```python
from build123d import *

# Parameters (mm, degrees)
BOSS_EXTRUDE6_DEPTH     = 13
SKETCH10_W              = 35
SKETCH10_H              = 50
BOSS_EXTRUDE7_DEPTH     = 200
BOSS_EXTRUDE8_DEPTH     = 13
BOSS_EXTRUDE10_DEPTH    = 200
FILLET2_R               = 0.2
FILLET3_R               = 0.2
SKETCH13_W              = 69.491392083
SKETCH13_H              = 95.024424652
SKETCH13_W_2            = 70.992171295
SKETCH13_H_2            = 120
CUT_EXTRUDE1_DEPTH      = 40
CUT_EXTRUDE1_DEPTH_BACK = 40
FILLET4_R               = 2


with BuildPart() as part:
    # Sketch9 → Boss-Extrude6 (new body)
    with BuildSketch(Plane(origin=(54.235591649, 0, 0), x_dir=(1, 0, 0), z_dir=(0, 0, 1))):
        Polygon((26.684813292, -242.858935562), (22.210553706, -242.858935562), (18.123114185, -244.678780887), (15.129250155, -248.003803746), (13.746627905, -252.259077482), (14.214315384, -256.708826606), (16.451445177, -260.583649071), (20.07119722, -263.213552871), (24.447683499, -264.143803746), (28.824169779, -263.213552871), (32.443921821, -260.583649071), (34.681051615, -256.708826606), (35.148739093, -252.259077482), (33.766116844, -248.003803746), (30.772252814, -244.678780887), align=None)
    extrude(amount=BOSS_EXTRUDE6_DEPTH)

    # Sketch10 → Boss-Extrude7 (add)
    with BuildSketch(Plane.XY.offset(13)):
        with Locations((78.683275149, -253.383803746)):
            Rectangle(SKETCH10_W, SKETCH10_H)
    extrude(amount=BOSS_EXTRUDE7_DEPTH)

    # Sketch11 → Boss-Extrude8 (add)
    with BuildSketch(Plane.XY.offset(213)):
        Polygon((78.683275149, -264.143803746), (83.059761428, -263.213552871), (86.679513471, -260.583649071), (88.916643264, -256.708826606), (89.384330743, -252.259077482), (88.001708493, -248.003803746), (85.007844463, -244.678780887), (80.920404942, -242.858935562), (76.446145356, -242.858935562), (72.358705834, -244.678780887), (69.364841804, -248.003803746), (67.982219555, -252.259077482), (68.449907033, -256.708826606), (70.687036827, -260.583649071), (74.306788869, -263.213552871), align=None)
    extrude(amount=BOSS_EXTRUDE8_DEPTH)

    # Sketch12 → Boss-Extrude10 (add)
    with BuildSketch(Plane.XY.offset(213)):
        Polygon((99.546985742, -240.476339651), (99.546985742, -240.976339651), (96.183275149, -240.976339651), (96.183275149, -245.876341177), (99.546985742, -245.876341177), (99.546985742, -246.376341177), (101.738909258, -245.329800525), (101.738909258, -244.726339651), (97.997187134, -244.726339651), (97.496982691, -244.234356535), (97.496982691, -242.626350386), (97.99698111, -242.126341177), (101.738909258, -242.126341177), (101.738909258, -241.524181899), align=None)
    extrude(amount=-BOSS_EXTRUDE10_DEPTH)

    # Fillet2
    fillet2_edges = [part.edges().sort_by_distance(p)[0] for p in [
        (101.738909258, -241.524181899, 113),
        (101.738909258, -242.126341177, 113),
        (97.99698111, -242.126341177, 113),
        (97.496982691, -242.626350386, 113),
        (97.496982691, -244.234356535, 113),
        (97.997187134, -244.726339651, 113),
        (101.738909258, -245.329800525, 113),
    ]]
    fillet(fillet2_edges, radius=FILLET2_R)

    # Fillet3
    fillet3_edges = [part.edges().sort_by_distance(p)[0] for p in [
        (101.738909258, -244.726339651, 113),
    ]]
    fillet(fillet3_edges, radius=FILLET3_R)

    # Sketch13 → Cut-Extrude1 (cut, two sides)
    with BuildSketch(Plane(origin=(0, -240.976339651, 0), x_dir=(1, 0, 0), z_dir=(0, 1, 0))) as cut_extrude1_sk:
        with Locations((130.928971191, -51.487787674)):
            Rectangle(SKETCH13_W, SKETCH13_H)
        with Locations((131.679360797, -187)):
            Rectangle(SKETCH13_W_2, SKETCH13_H_2)
    extrude(amount=CUT_EXTRUDE1_DEPTH, mode=Mode.SUBTRACT)
    extrude(cut_extrude1_sk.sketch, amount=-CUT_EXTRUDE1_DEPTH_BACK, mode=Mode.SUBTRACT)

    # Fillet4
    fillet4_edges = [part.edges().sort_by_distance(p)[0] for p in [
        (96.183275149, -278.383803746, 113),
        (96.183275149, -228.383803746, 113),
        (61.183275149, -228.383803746, 113),
        (61.183275149, -278.383803746, 113),
    ]]
    fillet(fillet4_edges, radius=FILLET4_R)


solid = part.part
```
Here's how the part is built. I have some questions about the finished solid (model axes, mm). A direction names the side the tool comes from. Round coordinates to 2 decimals unless told otherwise and drop trailing zeros. Loops run counter-clockwise (first coordinate to the right, second up) from the corner with the lowest first, then second, coordinate; pieces in that order, holes last.
1. Suppose I cut it at B-B, the plane y = -235.5. Please give me the cut outline in (x, z), and give its area (3 significant figures).
Answers:
outline: (61.18, 13) - (96.18, 13) - (96.18, 213) - (61.18, 213) - close
area: 7,000 mm2
2. Will these pins go through, and if not, where does the flat tip stop? pin 1 (3 mm diameter, centred on x = 100, z = 112, fed in from -Y); pin 2 (3.5 mm diameter, centred on x = 77.5, z = 6, fed in from +Y); pin 3 (3.5 mm diameter, centred on x = 98.5, z = 115.5, fed in from +Y).
Answers:
pin 1: stops at y = -246.38
pin 2: stops at y = -242.86
pin 3: stops at y = -240.48
3. Suppose I cut it at A-A, the plane z = 26. Please give me the cut outline in (x, y).
Answers:
outline: (61.18, -276.38) arc R2 ccw to (63.18, -278.38) - (94.18, -278.38) arc R2 ccw to (96.18, -276.38) - (96.18, -230.38) arc R2 ccw to (94.18, -228.38) - (63.18, -228.38) arc R2 ccw to (61.18, -230.38) - close
4. If I drill on probe 1 along X at (y, z) = (-258.5, 13.5); probe 2 along Z at (x, y) = (93.5, -260); probe 3 along X at (y, z) = (-244, 122), over which ranges is the centre line in solid material (lowest first)?
Answers:
probe 1: x = 61.18 to 96.18
probe 2: z = 13 to 213
probe 3: x = 61.18 to 97.5
5. Thinking about a two-plate mould opening in Z: for faces 5 (the face through (78, -242, 213)), 6 (the face through (84.84, -261.92, 219.41)), 7 (the face through (79, -253, 0)), which applies, released by +Z, released by -Z, zero draft, split by the parting line, or undercut?
Answers:
face 5: released by +Z
face 6: zero draft
face 7: released by -Z
6. For faces 1 (the face through (84.84, -261.92, 6.41)), 2 (the face through (76.46, -263.67, 219.41)), 3 (the face through (88.703, -250.161, 219.409)), 4 (the face through (79, -242.859, 6)), which set-ups out of +Z, -Z, +X, -X, +Y, -Y let a thin tool reach every point of the face, with its end or its side?
Answers:
face 1: -Z, +X, -Y
face 2: +Z, -X, -Y
face 3: +Z, +X, +Y
face 4: -Z, +X, -X, +Y
